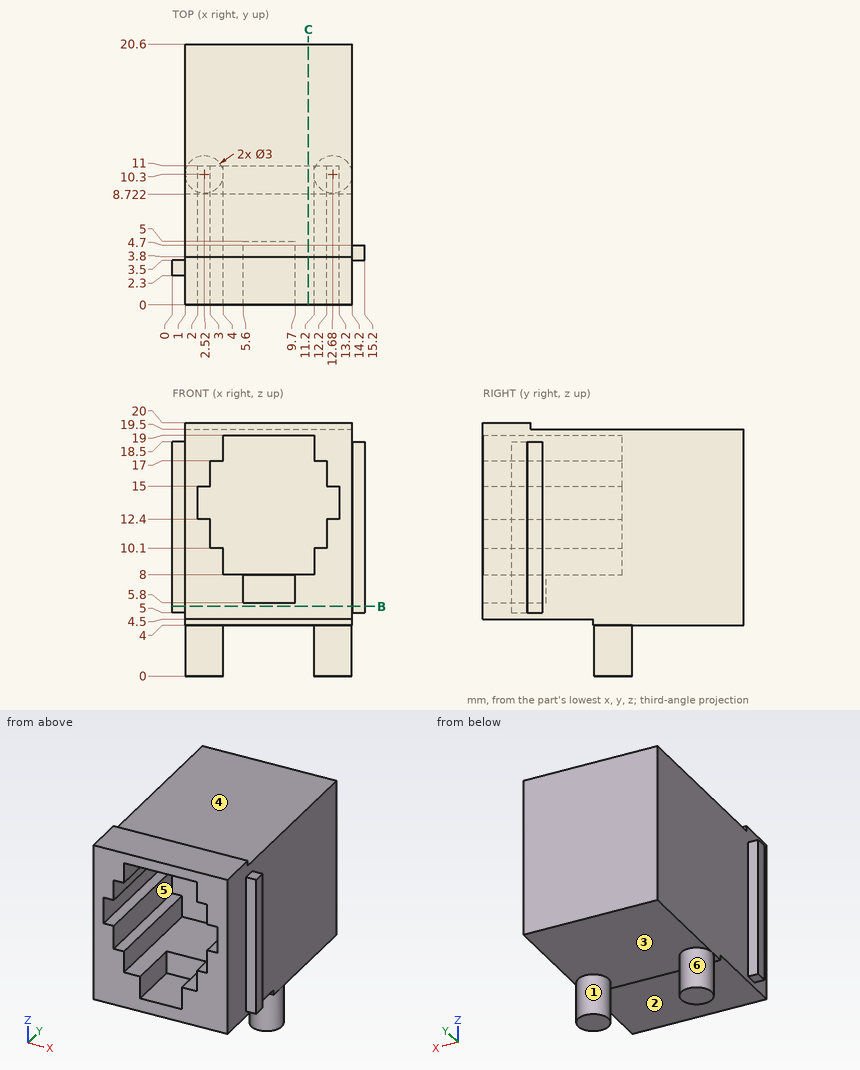
Print and shaded views of the part. All mm, measured from the part's lowest x, y and z. A direction names the side the tool comes from. Round coordinates to 2 decimals unless told otherwise and drop trailing zeros. Write each loop counter-clockwise with the first axis right and the second up, starting at its lowest first coordinate (ties: lowest second). Pieces come first, ordered by that corner, then holes.
Item 1: Which spindle directions (+Z, -Z, +X, -X, +Y, -Y) get a long thin tool onto all of the face, cutting with end or side? Do the marked faces 4, 5 and 6. Say none if no direction does.
Results:
face 4: +Z, +X, -X, +Y
face 5: -Y
face 6: -Z
Item 2: Probe L1, parallel to Z at x = 7, y = 7.75; L2, parallel to X at y = 4.75, z = 12.5; L3, parallel to X at y = 2.25, z = 18.5. List the from-to ranges inside material, lowest first.
Results:
L1: z = 4.5 to 8, 19 to 19.5
L2: x = 1 to 2, 13.2 to 14.2
L3: x = 1 to 4, 11.2 to 14.2
Item 3: Drop flat-ended pins along their axis: pin 1 Ø0.5 at (x, z) = (14.5, 10) entering from +Y; pin 2 Ø2 at (y, z) = (6, 8) entering from +X; pin 3 Ø0.5 at (x, y) = (0.5, 3) entering from +Z. Give the stop position or say it passes through.
Results:
pin 1: stops at y = 4.7
pin 2: stops at x = 14.2
pin 3: stops at z = 18.5
Item 4: Two-plate mould, pull along X, no slides. Class the marked faces 1, 2 and 3: +X half, -X half, draft (parallel to the pull), parting line (faces both ways), or undercut.
Results:
face 1: undercut
face 2: draft
face 3: undercut
Item 5: Cut at C-C, the plane x = 10.75. Give the cut face in (y, z).
Results:
outline: (0, 4.5) - (8.72, 4.5) - (8.72, 4) - (20.6, 4) - (20.6, 19.5) - (3.8, 19.5) - (3.8, 20) - (0, 20) - (0, 19) - (11, 19) - (11, 8) - (0, 8) - close
Item 6: Cut at B-B, the plane z = 5.5. Give the cut face in (x, y), plus the area to 3 significant figures.
Results:
outline: (0, 2.3) - (1, 2.3) - (1, 0) - (14.2, 0) - (14.2, 3.5) - (15.2, 3.5) - (15.2, 4.7) - (14.2, 4.7) - (14.2, 20.6) - (1, 20.6) - (1, 3.5) - (0, 3.5) - close
area: 274 mm2
